```python
from build123d import *

# Parameters (mm, degrees)
SKETCH1_W           = 172
SKETCH1_H           = 127
BOSS_EXTRUDE1_DEPTH = 1
BOSS_EXTRUDE2_DEPTH = 80
BOSS_EXTRUDE3_DEPTH = 68
SKETCH4_W           = 6
SKETCH4_H           = 8
SKETCH4_W_2         = 8
SKETCH4_H_2         = 6
BOSS_EXTRUDE4_DEPTH = 2
SKETCH5_W           = 42
SKETCH5_H           = 20
CUT_EXTRUDE1_DEPTH  = 10


with BuildPart() as part:
    # Sketch1 → Boss-Extrude1 (new body)
    with BuildSketch(Plane(origin=(0, 0, 0), x_dir=(1, 0, 0), z_dir=(0, 1, 0))):
        with Locations((86, 63.5)):
            Rectangle(SKETCH1_W, SKETCH1_H)
    extrude(amount=BOSS_EXTRUDE1_DEPTH)

    # Sketch1<3> → Boss-Extrude2 (add)
    with BuildSketch(Plane(origin=(0, 0, 0), x_dir=(1, 0, 0), z_dir=(0, 1, 0))):
        Polygon((-1, 128), (-1, 0), (0, 0), (0, 127), (172, 127), (172, 0), (173, 0), (173, 128), align=None)
    extrude(amount=BOSS_EXTRUDE2_DEPTH)

    # Sketch1<4> → Boss-Extrude3 (add)
    with BuildSketch(Plane(origin=(0, 0, 0), x_dir=(1, 0, 0), z_dir=(0, 1, 0))):
        Polygon((-1, 0), (-1, -1), (173, -1), (173, 0), (172, 0), (0, 0), align=None)
    extrude(amount=BOSS_EXTRUDE3_DEPTH)

    # Sketch4 → Boss-Extrude4 (add)
    with BuildSketch(Plane(origin=(0, 80, 0), x_dir=(1, 0, 0), z_dir=(0, 1, 0))):
        with Locations((2, 4)):
            Rectangle(SKETCH4_W, SKETCH4_H)
        with Locations((170, 4)):
            Rectangle(SKETCH4_W, SKETCH4_H)
        with Locations((86, 125)):
            Rectangle(SKETCH4_W_2, SKETCH4_H_2)
    extrude(amount=BOSS_EXTRUDE4_DEPTH)

    # Sketch5 → Cut-Extrude1 (cut)
    with BuildSketch(Plane.ZY.offset(1)):
        with Locations((-101, 70)):
            Rectangle(SKETCH5_W, SKETCH5_H)
    extrude(amount=-CUT_EXTRUDE1_DEPTH, mode=Mode.SUBTRACT)


solid = part.part
```
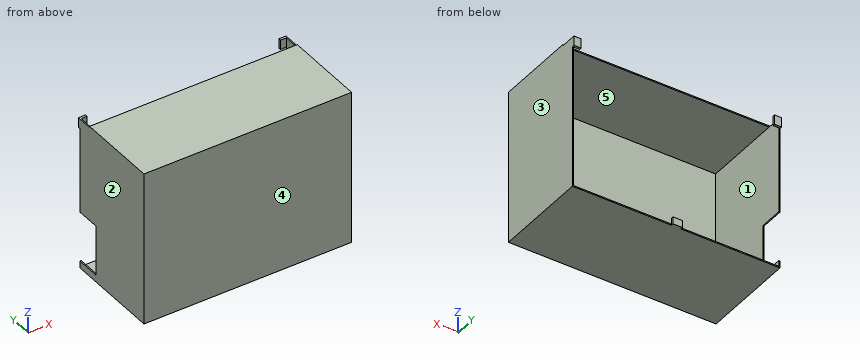
For this review, take the finished solid that the model builds, in its own axes (mm). Face numbers are marked on the shaded views. A direction names the side the tool comes from. Round coordinates to 2 decimals unless told otherwise and drop trailing zeros. Write each loop counter-clockwise with the first axis right and the second up, starting at its lowest first coordinate (ties: lowest second). Pieces come first, ordered by that corner, then holes.
1) Insertion check: pin 1 Ø10 at (x, z) = (123, -54) entering from -Y; pin 2 Ø1 at (x, z) = (114.5, -108.5) entering from +Y; pin 3 Ø3 at (x, y) = (171.5, 72) entering from +Z; pin 4 Ø0.6 at (x, y) = (1, 81) entering from -Z. Each pin has a flat end and moves straight along its axis. Give the tip position at first contact, or say it passes through.
Answer below:
pin 1: stops at y = 0
pin 2: stops at y = 1
pin 3: stops at z = 0
pin 4: stops at z = -8
2) For line 1 along Z through (x, y) = (23.5, 38); line 2 along X through (y, z) = (39, -36); line 3 along Y through (x, z) = (36, -111.5), list the stretches that pass through material, from the lowest coordinate up.
Answer below:
line 1: z = -128 to -127, 0 to 1
line 2: x = -1 to 0, 172 to 173
line 3: y = 0 to 1
3) Take a section at B-B on y = 65. Give the boundary of the cut face in (x, z), then the cut area to 3 significant figures.
Answer below:
outline: (-1, -128) - (173, -128) - (173, 1) - (-1, 1) - (-1, -80) - (0, -80) - (0, 0) - (172, 0) - (172, -127) - (0, -127) - (0, -122) - (-1, -122) - close
area: 560 mm2
4) Take a section at D-D on x = 128. Give the boundary of the cut face in (y, z).
Answer below:
outline: (0, -128) - (80, -128) - (80, -127) - (1, -127) - (1, 0) - (68, 0) - (68, 1) - (0, 1) - close
5) Take a section at A-A on z = -48. Give the boundary of the cut face in (x, y).
Answer below:
outline: (-1, 0) - (173, 0) - (173, 80) - (172, 80) - (172, 1) - (0, 1) - (0, 80) - (-1, 80) - close
6) Mouldability with a two-part tool opening along X and no side actions: class the marked faces 3, 4 and 5 as +X half, -X half, draft (parallel to the pull), parting line (faces both ways), or undercut.
Answer below:
face 3: +X half
face 4: draft
face 5: undercut
7) Machinability: for the marked faces 1 and 2, which of the approach directions +Z, -Z, +X, -X, +Y, -Y give a long, thin tool a straight path to every point of the face, cutting with its end or side? Answer none if there is none.
Answer below:
face 1: none
face 2: +Z, -Z, -X, +Y, -Y
8) Take a section at C-C on y = 31. Give the boundary of the cut face in (x, z).
Answer below:
outline: (-1, -128) - (173, -128) - (173, 1) - (-1, 1) - close; hole (0, -127) - (172, -127) - (172, 0) - (0, 0) - close
